For this review, take the finished solid that the model builds, in its own axes (mm). Give positions to 0.01 mm unless a question says otherwise; leave off trailing zeros. Order: outer loops, then holes, each group sorted by start corner. A loop starts at its lowest first (then second) coordinate and runs counter-clockwise, first axis right, second up. Notation, with made-up numbers: (5.25, 22.5) - (12.25, 22.5) arc R14 cw to (12.25, 38.5) - close; hole circle Ø10 at (24, 25). An arc over 180 degrees is marked (long way). Use a Markdown table: item, result. Add a question column.
1) Clearance check with a flat-ended pin moving along its axis: P1, Ø1, axis at x = 253.5, y = 2, coming from the -Z side. State where the tip first meets the part, or that it passes through.
2) We need section B-B on y = 1.6. Give the number of separate pieces and of enclosed holes in the cut face, then the cut area to 3 significant figures.
3) Wall thickness on L1, parallel to X at y = 1.3, z = 156; L2, parallel to Z at x = -395.7, y = 1.5; L3, parallel to X at y = 2.65, z = -200.5: over which ranges is each line inside the solid? List them lowest first.
4) We need section A-A on x = 385.5. Write out the cut boundary in (y, z).
```python
from build123d import *

# Parameters (mm, degrees)
BOSS_EXTRUDE2_DEPTH   = 3.26
SKETCH4_R             = 5
CUT_EXTRUDE7_DEPTH    = 10
SKETCH5_R             = 6
BEARING_HOLES_DEPTH   = 3.26
SKETCH7_R             = 3.5
CUT_EXTRUDE3_DEPTH    = 3.26
FRONT_HOLES_R         = 3.5
FRONT_HOLES_FET_DEPTH = 3.26
SKETCH10_R            = 3.500000002
SKETCH10_R_2          = 3.5
CUT_EXTRUDE5_DEPTH    = 3.26
CUT_EXTRUDE6_DEPTH    = 3.26
FILLET1_R             = 15
SKETCH13_R            = 5.588
CUT_EXTRUDE8_DEPTH    = 10
SKETCH14_R            = 2.75
CUT_EXTRUDE9_DEPTH    = 10


with BuildPart() as part:
    # Sketch1 → Boss-Extrude2 (new body)
    with BuildSketch(Plane(origin=(0, 0, 0), x_dir=(1, 0, 0), z_dir=(0, 1, 0))):
        Polygon((-165.1, 241.3), (-469.9, 241.3), (-469.9, -241.3), (-165.1, -241.3), (-165.1, -342.9), (165.1, -342.9), (165.1, -241.3), (469.9, -241.3), (469.9, 241.3), (165.1, 241.3), (165.1, 342.9), (-165.1, 342.9), align=None)
    extrude(amount=BOSS_EXTRUDE2_DEPTH)

    # Sketch4 → Cut-Extrude7 (cut)
    with BuildSketch(Plane(origin=(0, 3.26, 0), x_dir=(1, 0, 0), z_dir=(0, 1, 0))):
        with Locations(Location((-258.748000001, 93.5555, 0), (0, 0, 270))):
            Circle(SKETCH4_R)
        with Locations(Location((-128.573000001, 93.5555, 0), (0, 0, 270))):
            Circle(SKETCH4_R)
        with Locations(Location((1.601999999, 93.5555, 0), (0, 0, 270))):
            Circle(SKETCH4_R)
        with Locations(Location((131.776999999, 93.5555, 0), (0, 0, 270))):
            Circle(SKETCH4_R)
        with Locations(Location((261.951999999, 93.5555, 0), (0, 0, 270))):
            Circle(SKETCH4_R)
        with Locations(Location((256.172918992, -93.5555, 0), (0, 0, 270))):
            Circle(SKETCH4_R)
        with Locations(Location((125.997918992, -93.5555, 0), (0, 0, 270))):
            Circle(SKETCH4_R)
        with Locations(Location((-4.177081008, -93.5555, 0), (0, 0, 270))):
            Circle(SKETCH4_R)
        with Locations(Location((-134.352081008, -93.5555, 0), (0, 0, 270))):
            Circle(SKETCH4_R)
        with Locations(Location((-264.527081008, -93.5555, 0), (0, 0, 270))):
            Circle(SKETCH4_R)
    extrude(amount=-CUT_EXTRUDE7_DEPTH, mode=Mode.SUBTRACT)

    # Sketch5 → bearing holes (cut)
    with BuildSketch(Plane(origin=(0, 3.26, 0), x_dir=(1, 0, 0), z_dir=(0, 1, 0))):
        with Locations(Location((308.124918992, 211.3, 0), (0, 0, 270))):
            Circle(SKETCH5_R)
        with Locations(Location((403.824918992, 211.3, 0), (0, 0, 270))):
            Circle(SKETCH5_R)
        with Locations(Location((308.124918992, 100.0405, 0), (0, 0, 270))):
            Circle(SKETCH5_R)
        with Locations(Location((403.824918992, 100.0405, 0), (0, 0, 270))):
            Circle(SKETCH5_R)
        with Locations(Location((-395.7, -211.3, 0), (0, 0, 270))):
            Circle(SKETCH5_R)
        with Locations(Location((-300, -100.0405, 0), (0, 0, 270))):
            Circle(SKETCH5_R)
        with Locations(Location((-395.7, -100.0405, 0), (0, 0, 270))):
            Circle(SKETCH5_R)
        with Locations(Location((-300, -211.3, 0), (0, 0, 270))):
            Circle(SKETCH5_R)
        with Locations(Location((403.824918992, -105.2115, 0), (0, 0, 270))):
            Circle(SKETCH5_R)
        with Locations(Location((308.124918992, -105.2115, 0), (0, 0, 270))):
            Circle(SKETCH5_R)
        with Locations(Location((308.124918992, -211.3, 0), (0, 0, 270))):
            Circle(SKETCH5_R)
        with Locations(Location((403.824918992, -211.3, 0), (0, 0, 270))):
            Circle(SKETCH5_R)
        with Locations(Location((-300, 211.3, 0), (0, 0, 270))):
            Circle(SKETCH5_R)
        with Locations(Location((-395.7, 105.2115, 0), (0, 0, 270))):
            Circle(SKETCH5_R)
        with Locations(Location((-300, 105.2115, 0), (0, 0, 270))):
            Circle(SKETCH5_R)
        with Locations(Location((-395.7, 211.3, 0), (0, 0, 270))):
            Circle(SKETCH5_R)
    extrude(amount=-BEARING_HOLES_DEPTH, mode=Mode.SUBTRACT)

    # Sketch7 → Cut-Extrude3 (cut)
    with BuildSketch(Plane(origin=(0, 3.26, 0), x_dir=(1, 0, 0), z_dir=(0, 1, 0))):
        with Locations(Location((0, -223.64316, 0), (0, 0, 270))):
            Circle(SKETCH7_R)
        with Locations(Location((0, 223.64316, 0), (0, 0, 270))):
            Circle(SKETCH7_R)
        with Locations(Location((-88.9, -223.64316, 0), (0, 0, 270))):
            Circle(SKETCH7_R)
        with Locations(Location((-177.8, -223.64316, 0), (0, 0, 270))):
            Circle(SKETCH7_R)
        with Locations(Location((88.9, -223.64316, 0), (0, 0, 270))):
            Circle(SKETCH7_R)
        with Locations(Location((177.8, -223.64316, 0), (0, 0, 270))):
            Circle(SKETCH7_R)
        with Locations(Location((88.9, 223.64316, 0), (0, 0, 270))):
            Circle(SKETCH7_R)
        with Locations(Location((177.8, 223.64316, 0), (0, 0, 270))):
            Circle(SKETCH7_R)
        with Locations(Location((-88.9, 223.64316, 0), (0, 0, 270))):
            Circle(SKETCH7_R)
        with Locations(Location((-177.8, 223.64316, 0), (0, 0, 270))):
            Circle(SKETCH7_R)
    extrude(amount=-CUT_EXTRUDE3_DEPTH, mode=Mode.SUBTRACT)

    # front holes → front holes fet (cut)
    with BuildSketch(Plane(origin=(0, 3.26, 0), x_dir=(1, 0, 0), z_dir=(0, 1, 0))):
        with Locations(Location((459.075, 0.59516, 0), (0, 0, 270))):
            Circle(FRONT_HOLES_R)
        with Locations(Location((459.075, -99.40484, 0), (0, 0, 270))):
            Circle(FRONT_HOLES_R)
        with Locations(Location((459.075, -199.40484, 0), (0, 0, 270))):
            Circle(FRONT_HOLES_R)
        with Locations(Location((459.075, 100.59516, 0), (0, 0, 270))):
            Circle(FRONT_HOLES_R)
        with Locations(Location((459.075, 200.59516, 0), (0, 0, 270))):
            Circle(FRONT_HOLES_R)
        with Locations(Location((-459.075, 200.59516, 0), (0, 0, 270))):
            Circle(FRONT_HOLES_R)
        with Locations(Location((-459.075, 100.59516, 0), (0, 0, 270))):
            Circle(FRONT_HOLES_R)
        with Locations(Location((-459.075, -199.40484, 0), (0, 0, 270))):
            Circle(FRONT_HOLES_R)
        with Locations(Location((-459.075, -99.40484, 0), (0, 0, 270))):
            Circle(FRONT_HOLES_R)
        with Locations(Location((-459.075, 0.59516, 0), (0, 0, 270))):
            Circle(FRONT_HOLES_R)
    extrude(amount=-FRONT_HOLES_FET_DEPTH, mode=Mode.SUBTRACT)

    # Sketch10 → Cut-Extrude5 (cut)
    with BuildSketch(Plane(origin=(0, 3.26, 0), x_dir=(1, 0, 0), z_dir=(0, 1, 0))):
        with Locations(Location((-438.9, -223.64316, 0), (0, 0, 270))):
            Circle(SKETCH10_R)
        with Locations(Location((-438.9, 223.64316, 0), (0, 0, 270))):
            Circle(SKETCH10_R)
        with Locations(Location((438.9, 223.64316, 0), (0, 0, 270))):
            Circle(SKETCH10_R_2)
        with Locations(Location((438.9, -223.64316, 0), (0, 0, 270))):
            Circle(SKETCH10_R_2)
    extrude(amount=-CUT_EXTRUDE5_DEPTH, mode=Mode.SUBTRACT)

    # Sketch12 → Cut-Extrude6 (cut)
    with BuildSketch(Plane(origin=(0, 3.26, 0), x_dir=(1, 0, 0), z_dir=(0, 1, 0))):
        with BuildLine():
            Line((-426.702999083, 149.6355), (-436.550016189, 149.6355))
            ThreePointArc((-436.550016189, 149.6355), (-442.550016189, 155.6355), (-436.550016189, 161.6355))
            Line((-436.550016189, 161.6355), (-426.702999083, 161.6355))
            ThreePointArc((-426.702999083, 161.6355), (-420.702999083, 155.6355), (-426.702999083, 149.6355))
        make_face()
        with BuildLine():
            Line((-437.562081008, -149.6355), (-427.715063902, -149.6355))
            ThreePointArc((-427.715063902, -149.6355), (-421.715063902, -155.6355), (-427.715063902, -161.6355))
            Line((-427.715063902, -161.6355), (-437.562081008, -161.6355))
            ThreePointArc((-437.562081008, -161.6355), (-443.562081008, -155.6355), (-437.562081008, -149.6355))
        make_face()
        with BuildLine():
            Line((424.127918992, -149.6355), (433.974936098, -149.6355))
            ThreePointArc((433.974936098, -149.6355), (439.974936098, -155.6355), (433.974936098, -161.6355))
            Line((433.974936098, -161.6355), (424.127918992, -161.6355))
            ThreePointArc((424.127918992, -161.6355), (418.127918992, -155.6355), (424.127918992, -149.6355))
        make_face()
        with BuildLine():
            Line((434.987000917, 149.6355), (425.139983811, 149.6355))
            ThreePointArc((425.139983811, 149.6355), (419.139983811, 155.6355), (425.139983811, 161.6355))
            Line((425.139983811, 161.6355), (434.987000917, 161.6355))
            ThreePointArc((434.987000917, 161.6355), (440.987000917, 155.6355), (434.987000917, 149.6355))
        make_face()
    extrude(amount=-CUT_EXTRUDE6_DEPTH, mode=Mode.SUBTRACT)

    # Fillet1
    fillet1_edges = [part.edges().sort_by_distance(p)[0] for p in [
        (-165.1, 1.63, 241.3),
        (165.1, 1.63, 241.3),
        (165.1, 1.63, -241.3),
        (-165.1, 1.63, -241.3),
    ]]
    fillet(fillet1_edges, radius=FILLET1_R)

    # Sketch13 → Cut-Extrude8 (cut)
    with BuildSketch(Plane(origin=(0, 3.26, 0), x_dir=(1, 0, 0), z_dir=(0, 1, 0))):
        with Locations(Location((59, -258, 0), (0, 0, 270))):
            Circle(SKETCH13_R)
        with Locations(Location((0, -258, 0), (0, 0, 270))):
            Circle(SKETCH13_R)
        with Locations(Location((-59, -258, 0), (0, 0, 270))):
            Circle(SKETCH13_R)
        with Locations(Location((59, -288, 0), (0, 0, 270))):
            Circle(SKETCH13_R)
        with Locations(Location((0, -288, 0), (0, 0, 270))):
            Circle(SKETCH13_R)
        with Locations(Location((-59, -288, 0), (0, 0, 270))):
            Circle(SKETCH13_R)
        with Locations(Location((-59, 288, 0), (0, 0, 270))):
            Circle(SKETCH13_R)
        with Locations(Location((0, 288, 0), (0, 0, 270))):
            Circle(SKETCH13_R)
        with Locations(Location((59, 288, 0), (0, 0, 270))):
            Circle(SKETCH13_R)
        with Locations(Location((-59, 258, 0), (0, 0, 270))):
            Circle(SKETCH13_R)
        with Locations(Location((0, 258, 0), (0, 0, 270))):
            Circle(SKETCH13_R)
        with Locations(Location((59, 258, 0), (0, 0, 270))):
            Circle(SKETCH13_R)
    extrude(amount=-CUT_EXTRUDE8_DEPTH, mode=Mode.SUBTRACT)

    # Sketch14 → Cut-Extrude9 (cut)
    with BuildSketch(Plane(origin=(0, 3.26, 0), x_dir=(1, 0, 0), z_dir=(0, 1, 0))):
        with Locations(Location((135.1, 316.90316, 0), (0, 0, 270))):
            Circle(SKETCH14_R)
        with Locations(Location((135.1, 266.90316, 0), (0, 0, 270))):
            Circle(SKETCH14_R)
        with Locations(Location((-135.1, 266.90316, 0), (0, 0, 270))):
            Circle(SKETCH14_R)
        with Locations(Location((-135.1, 316.90316, 0), (0, 0, 270))):
            Circle(SKETCH14_R)
        with Locations(Location((135.1, -266.90316, 0), (0, 0, 270))):
            Circle(SKETCH14_R)
        with Locations(Location((135.1, -316.90316, 0), (0, 0, 270))):
            Circle(SKETCH14_R)
        with Locations(Location((-135.1, -316.90316, 0), (0, 0, 270))):
            Circle(SKETCH14_R)
        with Locations(Location((-135.1, -266.90316, 0), (0, 0, 270))):
            Circle(SKETCH14_R)
    extrude(amount=-CUT_EXTRUDE9_DEPTH, mode=Mode.SUBTRACT)


solid = part.part
```
Checked values:
| question | item | result |
|---|---|---|
| 1 | P1 | z = -241.3 |
| 2 | separate pieces | 1 |
| 2 | enclosed holes | 74 |
| 2 | area | 515,000 mm² |
| 3 | L1 | -469.9 to -443.55, -421.73 to 418.14, 439.96 to 469.9 |
| 3 | L2 | -241.3 to -217.3, -205.3 to -111.21, -99.21 to 94.04, 106.04 to 205.3, 217.3 to 241.3 |
| 3 | L3 | -469.9 to -462.57, -455.58 to 455.58, 462.57 to 469.9 |
| 4 | outline | (0, -241.3) - (3.26, -241.3) - (3.26, 241.3) - (0, 241.3) - close |
